Study the drawing (mm; zero at the part's minimum x, y, z) and answer. A direction names the side the tool comes from. Give positions to 0.01 mm unless a question says otherwise; leave off trailing zeros. Write each loop counter-clockwise with the first axis right and the second up, starting at its lowest first coordinate (ties: lowest second). Pieces come first, ordered by that corner, then holes. Notation, with made-up numbers: (67, 13.25) - (118, 13.25) arc R12 cw to (118, 26.25) - close; hole circle Ø6 at (29.25, 14.5). An arc over 180 degrees is marked (long way). Write each question's results on one line, items separated by ' | '. Start each with the question number.
Q1. Find the intervals of material crossed by probe 1 along Z at (x, y) = (39, 28); probe 2 along Z at (x, y) = (21, 8); probe 3 along X at (y, z) = (15.5, 24), in increasing order.
Q2. Section D-D (y = 5.5) is taken. Determine the outline of the cut face in (x, z), plus the area to 3 significant figures.
Q3. Section A-A (y = 18.5) is taken. Determine the outline of the cut face in (x, z).
Q4. Section C-C (x = 15) is taken. Determine the outline of the cut face in (y, z), plus the area to 3 significant figures.
Q5. Flat-ended cylindrical pins translate along their axes: pin 1 Ø15 at (x, y) = (46, 31) entering from +Z; pin 2 Ø10 at (y, z) = (28.5, 28) entering from -X; pin 3 Ø3 at (x, z) = (26, 12) entering from +Y. Find the tip coordinate at first contact, or state that the pin passes through.
Q6. For the marked faces 1 and 2, determine the directions among +Z, -Z, +X, -X, +Y, -Y from which every point of the face is accessible in a straight line to the end or side of a thin tool.
Q7. Section B-B (z = 19.5) is taken. Determine the outline of the cut face in (x, y), plus the area to 3 significant figures.
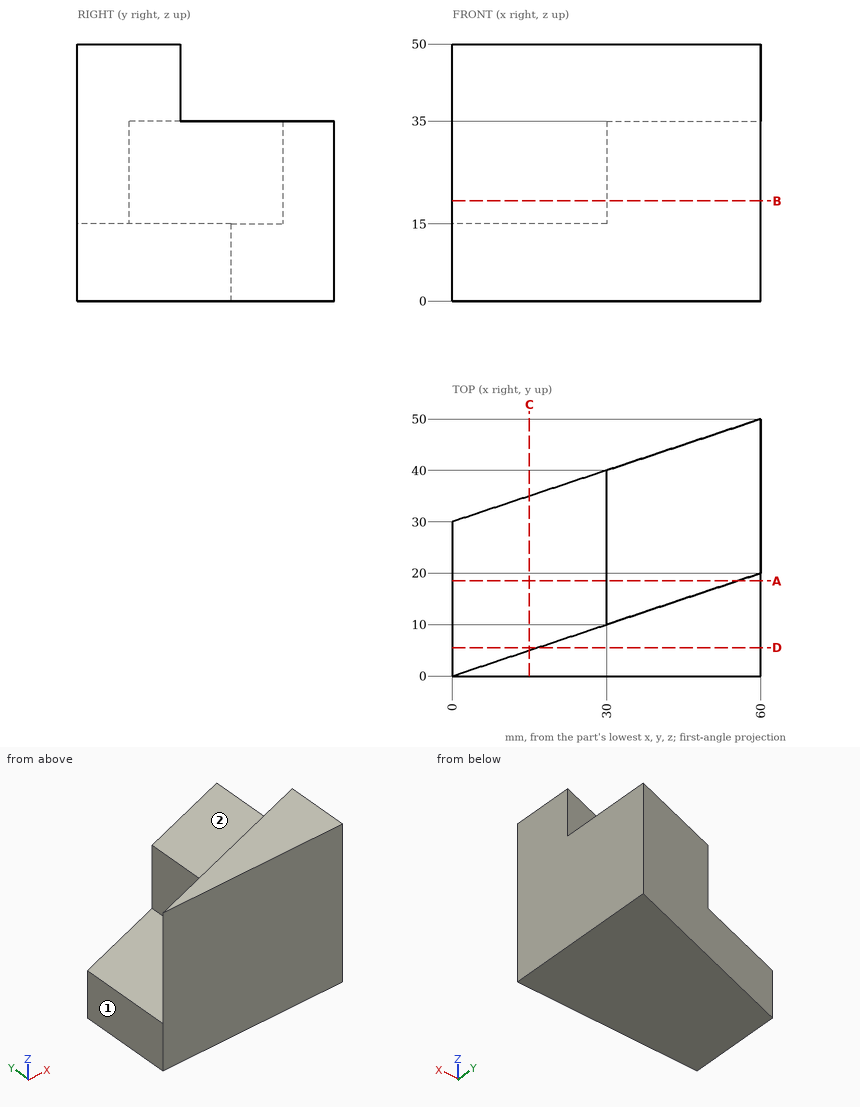
Answers below:
1) probe 1: z = 0 to 35 | probe 2: z = 0 to 15 | probe 3: x = 30 to 60
2) outline: (0, 0) - (60, 0) - (60, 50) - (16.5, 50) - (16.5, 15) - (0, 15) - close | area: 2,420 mm2
3) outline: (0, 0) - (60, 0) - (60, 50) - (55.5, 50) - (55.5, 35) - (30, 35) - (30, 15) - (0, 15) - close
4) outline: (0, 0) - (35, 0) - (35, 15) - (5, 15) - (5, 50) - (0, 50) - close | area: 700 mm2
5) pin 1: stops at z = 35 | pin 2: stops at x = 30 | pin 3: stops at y = 39.17
6) face 1: +Z, -Z, -X, +Y, -Y | face 2: +Z, -X, +Y
7) outline: (0, 0) - (60, 0) - (60, 50) - (30, 40) - (30, 10) - close | area: 1,500 mm2
